Part model, mm, in its own coordinate system. Face numbers are marked on the shaded views. A direction names the side the tool comes from. Round coordinates to 2 decimals unless told otherwise and drop trailing zeros. Order: outer loops, then holes, each group sorted by start corner. A loop starts at its lowest first (then second) coordinate and runs counter-clockwise, first axis right, second up. Notation, with made-up numbers: (18, 27.5) - (55, 27.5) arc R16 cw to (55, 50.5) - close; hole circle Ø1 at (72.25, -3.75). An arc over 180 degrees is marked (long way). Answer as a JSON object with one key per item and string values.
```python
from build123d import *

# Parameters (mm, degrees)
BOSS_EXTRUDE1_DEPTH = 10
SKETCH2_R           = 1.75
CUT_EXTRUDE1_DEPTH  = 10


with BuildPart() as part:
    # Sketch1 → Boss-Extrude1 (new, symmetric)
    with BuildSketch(Plane.XY):
        Polygon((0, 0), (18.4, 0), (18.4, 9.6), (4.2, 9.6), (4.2, 4.2), (14.2, 4.2), (14.2, 5.4), (5.4, 5.4), (5.4, 8.4), (17.2, 8.4), (17.2, 1.2), (1.2, 1.2), (1.2, 16), (0, 16), align=None)
    extrude(amount=BOSS_EXTRUDE1_DEPTH, both=True)

    # Sketch2 → Cut-Extrude1 (cut, symmetric)
    with BuildSketch(Plane(origin=(1.2, 0, 0), x_dir=(0, 0, -1), z_dir=(1, 0, 0))):
        with Locations((-6, 12)):
            Circle(SKETCH2_R)
        with Locations((6, 12)):
            Circle(SKETCH2_R)
    extrude(amount=CUT_EXTRUDE1_DEPTH, both=True, mode=Mode.SUBTRACT)


solid = part.part
```
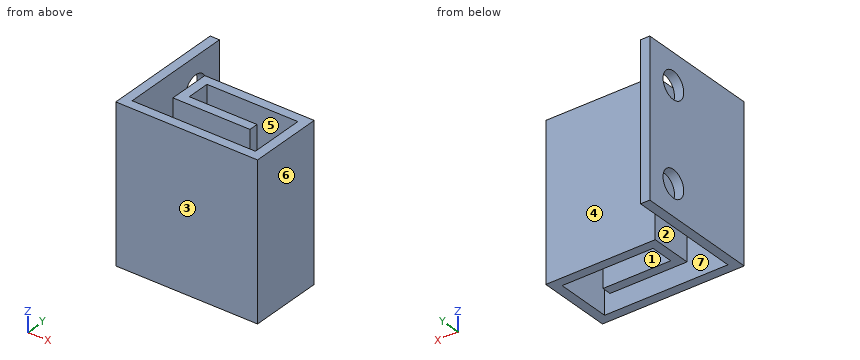
Item 1: Cut at A-A (y = 12). Write the cut outline in (x, z).
Taken from the geometry:
{"outline": "(0, -10) - (1.2, -10) - (1.2, -7.75) - (0, -7.75) - close; (0, -4.25) - (1.2, -4.25) - (1.2, 4.25) - (0, 4.25) - close; (0, 7.75) - (1.2, 7.75) - (1.2, 10) - (0, 10) - close"}
Item 2: Probe L1, parallel to Y at x = 8.5, z = 2; L2, parallel to X at y = 8.25, z = -1; L3, parallel to Y at x = 0.4, z = 6. List the from-to ranges inside material, lowest first. Write a range as from..to.
Taken from the geometry:
{"L1": "0..1.2, 4.2..5.4, 8.4..9.6", "L2": "0..1.2, 4.2..5.4, 17.2..18.4", "L3": "0..10.25, 13.75..16"}
Item 3: Tool access for the marked faces 1, 2 and 3: list every direction of +Z, -Z, +X, -X, +Y, -Y with a clear straight run to the whole face (end or side of a thin tool).
Taken from the geometry:
{"face 1": "+Z, -Z", "face 2": "+Z, -Z, +Y", "face 3": "+Z, -Z, +X, -X, -Y"}
Item 4: Cut at C-C (y = 2.25). Write the cut outline in (x, z).
Taken from the geometry:
{"outline": "(0, -10) - (1.2, -10) - (1.2, 10) - (0, 10) - close; (17.2, -10) - (18.4, -10) - (18.4, 10) - (17.2, 10) - close"}
Item 5: Cut at D-D (z = -6). Write the cut outline in (x, y), plus the area to 3 significant figures.
Taken from the geometry:
{"outline": "(0, 0) - (18.4, 0) - (18.4, 9.6) - (4.2, 9.6) - (4.2, 4.2) - (14.2, 4.2) - (14.2, 5.4) - (5.4, 5.4) - (5.4, 8.4) - (17.2, 8.4) - (17.2, 1.2) - (1.2, 1.2) - (1.2, 10.25) - (0, 10.25) - close; (0, 13.75) - (1.2, 13.75) - (1.2, 16) - (0, 16) - close", "area": "76.9 mm2"}
Item 6: Two-plate mould, pull along X, no slides. Class the marked faces 4, 5, 6 and 7: pulls with the +X half, pulls with the -X half, needs draft (parallel to the pull), parting line crosses it, or undercut.
Taken from the geometry:
{"face 4": "needs draft", "face 5": "undercut", "face 6": "pulls with the +X half", "face 7": "undercut"}
Item 7: Cut at B-B (x = 6). Write the cut outline in (y, z), plus the area to 3 significant figures.
Taken from the geometry:
{"outline": "(0, -10) - (1.2, -10) - (1.2, 10) - (0, 10) - close; (4.2, -10) - (5.4, -10) - (5.4, 10) - (4.2, 10) - close; (8.4, -10) - (9.6, -10) - (9.6, 10) - (8.4, 10) - close", "area": "72.0 mm2"}
Item 8: Drop flat-ended pins along their axis: P1, Ø7, axis at x = 10.5, z = -3.5, coming from the +Y side; P2, Ø3, axis at y = 12, z = 6, coming from the +X side; P3, Ø2, axis at x = 2.5, z = -5.5, coming from the +Y side. Give the stop position or say it passes through.
Taken from the geometry:
{"P1": "y = 9.6", "P2": "through", "P3": "y = 1.2"}
